Autodesk Inventor part; units mm, degrees
ref_plane "YZ Plane" through (0, 0, 0) normal (1, 0, 0) x (0, 1, 0)
ref_plane "XZ Plane" through (0, 0, 0) normal (0, 1, 0) x (-1, 0, 0)
ref_plane "XY Plane" through (0, 0, 0) normal (0, 0, 1) x (1, 0, 0)
sketch "Sketch1" plane through (0, 0, 0) normal (1, 0, 0) x (0, 1, 0)
  circle A0 centre (0, 0) radius 25.4
  line L0 (0, -25.4) -> (-21.997, -12.7)
  line L1 (-21.997, -12.7) -> (-21.997, 12.7)
  line L2 (-21.997, 12.7) -> (0, 25.4)
  line L3 (0, 25.4) -> (21.997, 12.7)
  line L4 (21.997, 12.7) -> (21.997, -12.7)
  line L5 (21.997, -12.7) -> (0, -25.4)
  dimension "d0" = 50.8
extrude "Extrusion1" add sketch "Sketch1" along normal blind 76.2 contours L4 L5 L0 L1 L2 L3
sketch "Sketch2" plane through (0, 0, 0) normal (0, 1, 0) x (-1, 0, 0)
  line L0 (0, 25.4259) -> (-25.4, 25.4)
  line L1 (0, 25.4) -> (-76.2, 25.4)
  line L2 (-25.4, 25.4) -> (-79.2265, -28.5365)
  line L3 (-79.2265, -28.5365) -> (-79.2893, 33.005)
  line L4 (-79.2893, 33.005) -> (-25.4, 25.4)
  point P0 (0, 0)
  dimension "d3" = 25.4
  dimension "d4" = 76.2
  dimension "d5" = 135
extrude "Extrusion2" cut sketch "Sketch2" along normal mid plane 76.2
CAD build for the part. Positions are in the model's coordinates, mm. Round coordinates to 2 decimals unless told otherwise and drop trailing zeros. Order: outer loops, then holes, each group sorted by start corner. A loop starts at its lowest first (then second) coordinate and runs counter-clockwise, first axis right, second up. Notation, with made-up numbers: (-16, -19.75) - (32, -19.75) arc R13 ccw to (32, 2.25) - close; hole circle Ø6 at (82.5, -16). An arc over 180 degrees is marked (long way). Answer as CSV lines item,"result". Start each with the question number.
1. Saw through at C-C, the plane y = 11. Write the cut outline in (x, z).
2. Saw through at A-A, the plane x = 13. Write the cut outline in (y, z), and give its area (3 significant figures).
3. Saw through at D-D, the plane x = 48. Write the cut outline in (y, z), and give its area (3 significant figures).
4. Drill centre lines: L1, parallel to X at y = -2.5, z = 9.5; L2, parallel to Z at x = 50.5, y = -13.5; L3, parallel to Z at x = 64.5, y = -1. Where is each one in solid material? Low to high. Write a range as [from, to].
5. Saw through at B-B, the plane z = 5.5. Write the cut outline in (x, y), and give its area (3 significant figures).
6. Pin check, flat tips, straight feed: pin 1 (2 mm diameter, centred on x = 39, y = -12.5, fed in from +Z); pin 2 (10 mm diameter, centred on x = 34.5, y = -14, fed in from -Z); pin 3 (1 mm diameter, centred on x = 29.5, y = 17, fed in from -Z); pin 4 (10 mm diameter, centred on x = 53, z = 6.5, fed in from +Y). Stop position of each tip, or through.
Model answer:
1,outline,"(0, -19.05) - (69.76, -19.05) - (31.74, 19.05) - (0, 19.05) - close"
2,outline,"(-22, -12.7) - (0, -25.4) - (22, -12.7) - (22, 12.7) - (0, 25.4) - (-22, 12.7) - close"
2,area,"1,680 mm²"
3,outline,"(-22, -12.7) - (0, -25.4) - (22, -12.7) - (22, 2.75) - (-22, 2.75) - close"
3,area,"959 mm²"
4,L1,"x = [0, 41.27]"
4,L2,"z = [-17.61, 0.25]"
4,L3,"z = [-24.82, -13.78]"
5,outline,"(0, -22) - (45.26, -22) - (45.26, 22) - (0, 22) - close"
5,area,"1,990 mm²"
6,pin 1,"stops at z = 12.77"
6,pin 2,"stops at z = -20.2"
6,pin 3,"stops at z = -15.87"
6,pin 4,"passes through"
